The listing builds one solid part. Answer for the finished solid, in the listing's coordinates (mm). Coordinates: 2 decimals unless noted, no trailing zeros. Loops run counter-clockwise (first coordinate to the right, second up) from the corner with the lowest first, then second, coordinate; pieces in that order, holes last. Notation, with made-up numbers: M -38.75,50 L -21.75,50 A13 ccw -21.75,54 Z; hole C 35.25,84 d1. An arc over 180 degrees is marked long. Answer as CSV lines item,"result". Start each with the question number.
```python
from build123d import *

# Parameters (mm, degrees)
SKETCH015_R      = 150
EXTRUDE011_DEPTH = 20
SKETCH014_W      = 820
SKETCH014_H      = 820
EXTRUDE009_DEPTH = 20


with BuildPart() as extrude013:
    # Sketch015 (on Face6 of Extrude009) → Extrude011 (new body)
    with BuildSketch(Plane.XY.offset(370)):
        Circle(SKETCH015_R)
    extrude(amount=-EXTRUDE011_DEPTH)


with BuildPart() as cut006:
    # Sketch014 (on Face8 of Extrude) → Extrude009 (new body)
    with BuildSketch(Plane.XY.offset(350)):
        Rectangle(SKETCH014_W, SKETCH014_H)
    extrude(amount=EXTRUDE009_DEPTH)

    # Cut006: cut Extrude013
    add(extrude013.part, mode=Mode.SUBTRACT)


solid = cut006.part
```
Item 1: Section A-A on y = 0 is taken. Determine the outline of the cut face in (x, z), then the cut area to 3 significant figures.
Item 2: For a pull along Y with two mould halves and no side action, classify faces 1 (the face through (-6, 410, 360)), 2 (the face through (-19.527, 148.724, 360.14)), 3 (the face through (410, -6, 360)) as pulls with the +Y half, pulls with the -Y half, needs draft (parallel to the pull), parting line crosses it, or undercut.
Item 3: Section C-C on z = 363 is taken. Determine the outline of the cut face in (x, y).
Item 4: Consider line 1 (Y direction, x = 0, z = 364); line 2 (X direction, y = 5, z = 351.5); line 3 (X direction, y = -74.5, z = 364). Determine where each line is inside the solid, lowest interval first.
Results are:
1,outline,"M -410,350 L -150,350 L -150,370 L -410,370 Z; M 150,350 L 410,350 L 410,370 L 150,370 Z"
1,area,"10,400 mm²"
2,face 1,"pulls with the +Y half"
2,face 2,"undercut"
2,face 3,"needs draft"
3,outline,"M -410,-410 L 410,-410 L 410,410 L -410,410 Z; hole C 0,0 d300"
4,line 1,"-410 to -150, 150 to 410"
4,line 2,"-410 to -149.92, 149.92 to 410"
4,line 3,"-410 to -130.19, 130.19 to 410"
